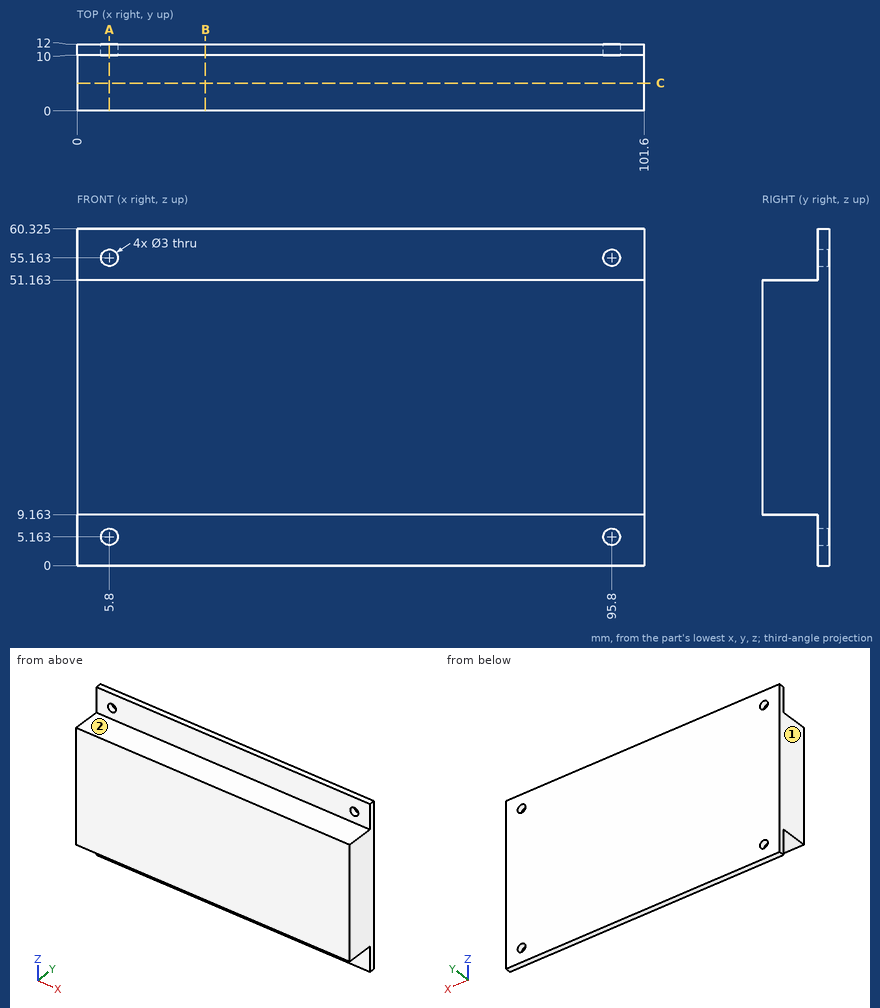
Geometry check sheet. Reference: drawing and pictorial views, mm from the part's lowest x, y, z. A direction names the side the tool comes from. Round coordinates to 2 decimals unless told otherwise and drop trailing zeros. Loops run counter-clockwise (first coordinate to the right, second up) from the corner with the lowest first, then second, coordinate; pieces in that order, holes last. Notation, with made-up numbers: (19, 71) - (39, 71) arc R29 ccw to (39, 102) - close; hole circle Ø4 at (-31, 24.5). An arc over 180 degrees is marked (long way). Write item = value, one per line. Start each with the question number.
Q1. Access from +Z, -Z, +X, -X, +Y, -Y to the whole of each face (thin tool, end or side, straight path). Record for the marked faces 1 and 2.
Q2. Thickness scan on L1, parallel to Z at x = 95.8, y = 11.1 (1 decimal); L2, parallel to Y at x = 63, z = 53.5; L3, parallel to Z at x = 52.5, y = 5. Record the ranges inside material, lowest first.
Q3. Section check B-B (x = 23). Record the boundary of the cut face in (y, z) (1 decimal).
Q4. Section check A-A (x = 5.8). Record the boundary of the cut face in (y, z) (1 decimal), plus the area to 3 significant figures.
Q5. Section check C-C (y = 5). Record the boundary of the cut face in (x, z).
Q6. Depth check by flat-ended pin: P1, Ø2.5, axis at x = 61.5, z = 57, coming from the -Y side; P2, Ø1, axis at x = 75.5, y = 9, coming from the +Z side; P3, Ø2, axis at x = 54, y = 3, coming from the -Z side. Enter the tip coordinate at first touch or a pass-through.
Derived:
q1.face_1 = +Z, -Z, -X, +Y, -Y
q1.face_2 = +Z, +X, -X, -Y
q2.L1 = 0 to 3.7, 6.7 to 53.7, 56.7 to 60.3
q2.L2 = 10 to 12
q2.L3 = 9.16 to 51.16
q3.outline = (0, 9.2) - (10, 9.2) - (10, 0) - (12, 0) - (12, 60.3) - (10, 60.3) - (10, 51.2) - (0, 51.2) - close
q4.outline = (0, 9.2) - (10, 9.2) - (10, 6.7) - (12, 6.7) - (12, 53.7) - (10, 53.7) - (10, 51.2) - (0, 51.2) - close; (10, 0) - (12, 0) - (12, 3.7) - (10, 3.7) - close; (10, 56.7) - (12, 56.7) - (12, 60.3) - (10, 60.3) - close
q4.area = 529 mm^2
q5.outline = (0, 9.16) - (101.6, 9.16) - (101.6, 51.16) - (0, 51.16) - close
q6.P1 = 10
q6.P2 = 51.16
q6.P3 = 9.16
